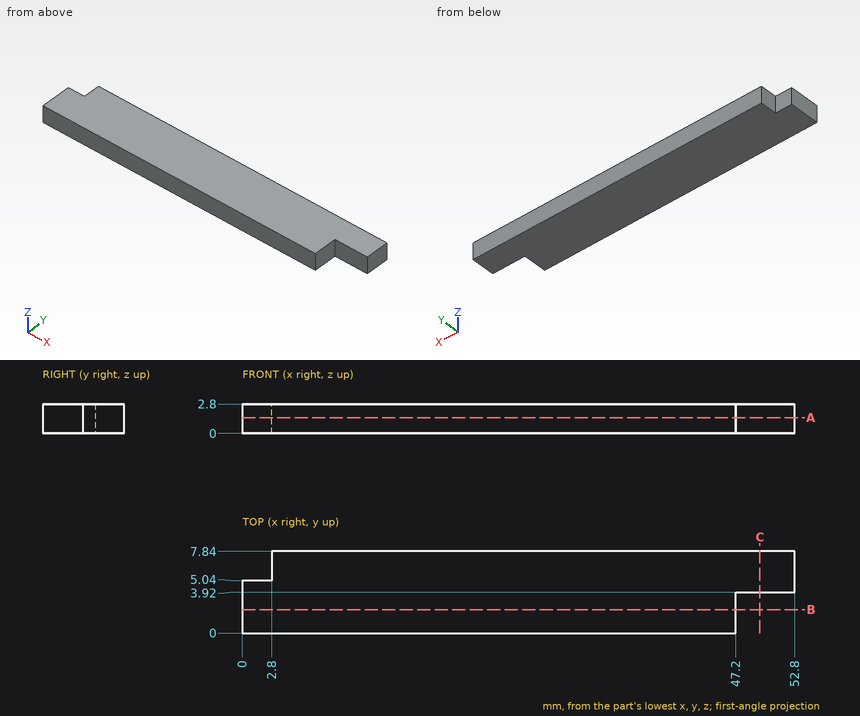
Answer from the drawing. Dimensions are ordinates in mm from the lowest x, y and z of the part. Give positions to 0.01 mm unless a question says otherwise; leave off trailing zeros. Write each loop counter-clockwise with the first axis right and the second up, starting at its lowest first coordinate (ties: lowest second). Pieces come first, ordered by that corner, then holes. Notation, with made-up numbers: (47.5, -18) - (74.5, -18) arc R5 ccw to (74.5, -10) - close; hole circle Ø8 at (78, -5.5). An arc over 180 degrees is marked (long way). One line per item, written item: value. Start each with the question number.
1. Find section A-A (z = 1.5). Write down the section's boundary in (x, y), then the cut area to 3 significant figures.
2. Find section B-B (y = 2.25). Write down the section's boundary in (x, z).
3. Given pin 1 (1 mm diameter, centred on y = 3, z = 1, fed in from +X), flat-ended and moving along its own axis, determine where the tip first touches the part or whether it passes through.
4. Consider probe 1 along X at (y, z) = (2.5, 1.9); probe 2 along Y at (x, z) = (49, 1.8); probe 3 along X at (y, z) = (7, 1.5). Determine where each line is inside the solid, lowest interval first.
5. Find section C-C (x = 49.5). Write down the section's boundary in (y, z).
Geometry results:
1. outline: (0, 0) - (47.2, 0) - (47.2, 3.92) - (52.8, 3.92) - (52.8, 7.84) - (2.8, 7.84) - (2.8, 5.04) - (0, 5.04) - close
1. area: 384 mm2
2. outline: (0, 0) - (47.2, 0) - (47.2, 2.8) - (0, 2.8) - close
3. pin 1: x = 47.2
4. probe 1: 0 to 47.2
4. probe 2: 3.92 to 7.84
4. probe 3: 2.8 to 52.8
5. outline: (3.92, 0) - (7.84, 0) - (7.84, 2.8) - (3.92, 2.8) - close
